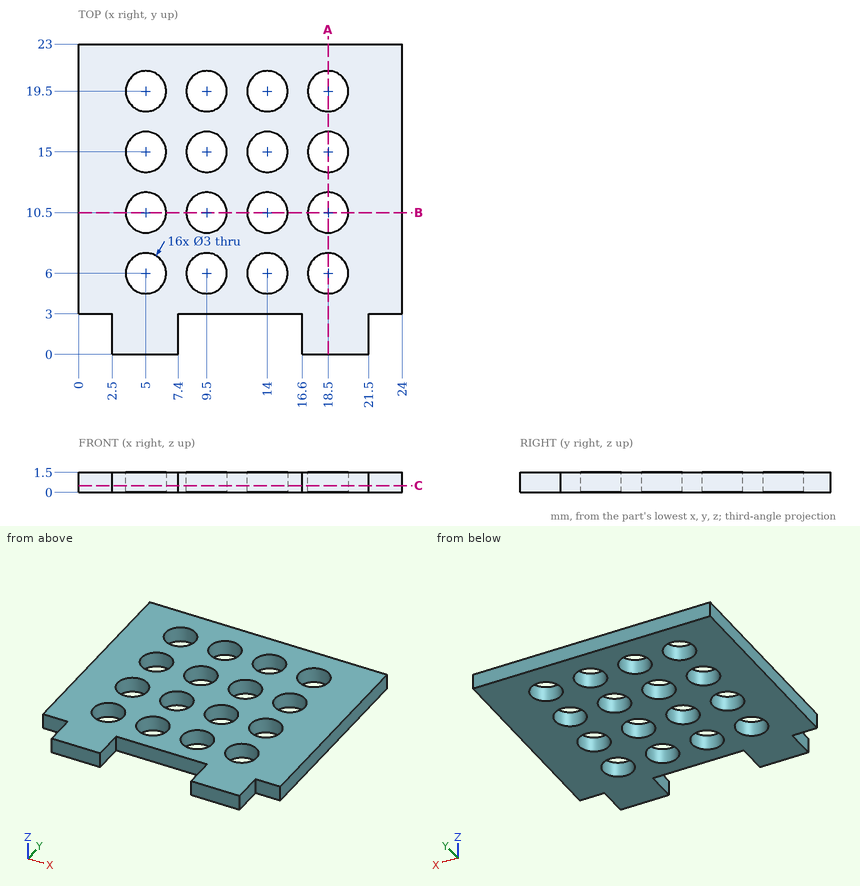
Geometry check sheet. Reference: drawing and pictorial views, mm from the part's lowest x, y, z. Round coordinates to 2 decimals unless told otherwise and drop trailing zeros. Loops run counter-clockwise (first coordinate to the right, second up) from the corner with the lowest first, then second, coordinate; pieces in that order, holes last. Notation, with made-up numbers: (41, 26) - (55, 26) arc R27 ccw to (55, 50) - close; hole circle Ø10 at (77.25, 61). An arc over 180 degrees is marked (long way). Use a Markdown table: item, result.
Q1. Cross-section at B-B on y = 10.5. Record the cut outline in (x, z).
Solutions:
| item | result |
|---|---|
| outline | (0, 0) - (3.5, 0) - (3.5, 1.5) - (0, 1.5) - close; (6.5, 0) - (8, 0) - (8, 1.5) - (6.5, 1.5) - close; (11, 0) - (12.5, 0) - (12.5, 1.5) - (11, 1.5) - close; (15.5, 0) - (17, 0) - (17, 1.5) - (15.5, 1.5) - close; (20, 0) - (24, 0) - (24, 1.5) - (20, 1.5) - close |
Q2. Cross-section at A-A on x = 18.5. Record the cut outline in (y, z).
Solutions:
| item | result |
|---|---|
| outline | (0, 0) - (4.5, 0) - (4.5, 1.5) - (0, 1.5) - close; (7.5, 0) - (9, 0) - (9, 1.5) - (7.5, 1.5) - close; (12, 0) - (13.5, 0) - (13.5, 1.5) - (12, 1.5) - close; (16.5, 0) - (18, 0) - (18, 1.5) - (16.5, 1.5) - close; (21, 0) - (23, 0) - (23, 1.5) - (21, 1.5) - close |
Q3. Cross-section at C-C on z = 0.5. State how many separate pieces and enclosed holes the cut face has, plus the area to 3 significant figures.
Solutions:
| item | result |
|---|---|
| separate pieces | 1 |
| enclosed holes | 16 |
| area | 396 mm2 |
Q4. Go/stop test with flat-tipped pins: P1, Ø0.8, axis at x = 1, z = 0.5, coming from the -Y side; P2, Ø2.5, axis at x = 5, y = 10.5, coming from the -Z side; P3, Ø0.8, axis at y = 1, z = 0.5, coming from the -X side. Record where each tip stops, or that it passes through.
Solutions:
| item | result |
|---|---|
| P1 | stops at y = 3 |
| P2 | passes through |
| P3 | stops at x = 2.5 |
Q5. Material ranges on line 1 (Y direction, x = 18.5, z = 0.55); line 2 (Y direction, x = 15.25, z = 1.25); line 3 (X direction, y = 18.75, z = 0.35), recorded low to high.
Solutions:
| item | result |
|---|---|
| line 1 | y = 0 to 4.5, 7.5 to 9, 12 to 13.5, 16.5 to 18, 21 to 23 |
| line 2 | y = 3 to 5.17, 6.83 to 9.67, 11.33 to 14.17, 15.83 to 18.67, 20.33 to 23 |
| line 3 | x = 0 to 3.7, 6.3 to 8.2, 10.8 to 12.7, 15.3 to 17.2, 19.8 to 24 |
